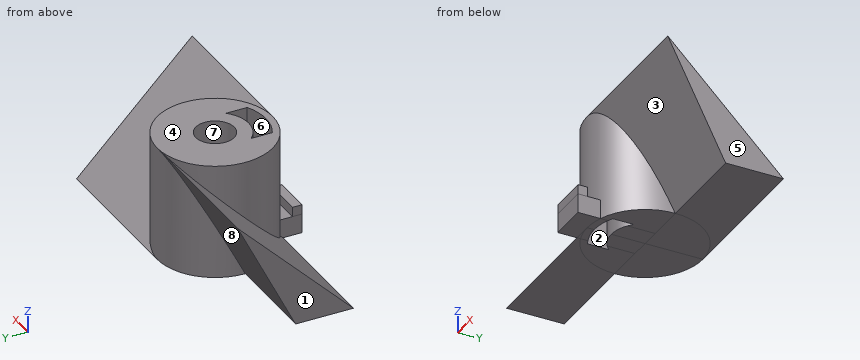
from build123d import *
from build123d import SkipClean  # not in build123d's __all__

# Parameters (mm, degrees)
F0_R      = 7.62
F1_DEPTH  = 15.24
F3_DEPTH  = 20.32
F5_COUNT  = 2
F6_W      = 5.0799995622
F6_H      = 2.54
F7_DEPTH  = 10.16
F8_W      = 5.0799995622
F8_H      = 1.27
F9_DEPTH  = 1.27
F10_R     = 2.54
F11_DEPTH = 13.97
F13_DEPTH = 25.4


with BuildPart() as f1:
    # F0 (on Top) → F1 (new body)
    with BuildSketch(Plane.XY):
        Circle(F0_R)
    extrude(amount=F1_DEPTH)



with BuildPart() as f3:
    # F2 (on Right) → F3 (new body)
    with BuildSketch(Plane.YZ):
        Polygon((-7.62, 15.24), (0, 0), (7.62, 0), align=None)
    extrude(amount=F3_DEPTH)


with BuildPart() as f1_1:
    add(f1.part, clean=False)

    with SkipClean():  # cleaning this boolean's faces spoils the solid; the shape is the same uncleaned
        add(f3.part)  # F5 merges F3
    # F5: F3 ×2 about axis
    f5_axis = Axis((0, 0, 17.5851359963), (0, 0, 1))
    with SkipClean():  # cleaning this boolean's faces spoils the solid; the shape is the same uncleaned
        for i in range(1, F5_COUNT):
            add(f3.part.rotate(f5_axis, i * 360 / F5_COUNT), clean=False)

    # F6 (on Front) → F7 (join)
    with BuildSketch(Plane.XZ):
        with Locations((0, 1.27)):
            Rectangle(F6_W, F6_H)
    with SkipClean():  # cleaning this boolean's faces spoils the solid; the shape is the same uncleaned
        extrude(amount=F7_DEPTH)

    # F8 (on face) → F9 (join)
    with BuildSketch(Plane.XY.offset(2.54)):
        with Locations((0, -9.525)):
            Rectangle(F8_W, F8_H)
    with SkipClean():  # cleaning this boolean's faces spoils the solid; the shape is the same uncleaned
        extrude(amount=F9_DEPTH)

    # F10 (on face) → F11 (cut)
    with BuildSketch(Plane.XY.offset(15.24)):
        Circle(F10_R)
    with SkipClean():  # cleaning this boolean's faces spoils the solid; the shape is the same uncleaned
        extrude(amount=-F11_DEPTH, mode=Mode.SUBTRACT)

    # F12 (on face) → F13 (cut)
    with BuildSketch(Plane.XY.offset(15.24)):
        with BuildLine():
            ThreePointArc((3.175, -3.1108519733), (0, -4.445), (-3.175, -3.1108519733))
            Line((-3.175, -3.1108519733), (-3.175, -5.9048519733))
            ThreePointArc((-3.175, -5.9048519733), (0, -6.7043196394), (3.175, -5.9048519733))
            Line((3.175, -5.9048519733), (3.175, -3.1108519733))
        make_face()
    with SkipClean():  # cleaning this boolean's faces spoils the solid; the shape is the same uncleaned
        extrude(amount=-F13_DEPTH, mode=Mode.SUBTRACT)


solid = f1_1.part
Work out the finished part from the listing and answer in its coordinate system (mm). Face numbers are marked on the shaded views. A direction names the side the tool comes from. Round coordinates to 2 decimals unless told otherwise and drop trailing zeros. Loops run counter-clockwise (first coordinate to the right, second up) from the corner with the lowest first, then second, coordinate; pieces in that order, holes last. Notation, with made-up numbers: M 80.5,-24.75 L 118.5,-24.75 A21 cw 118.5,7.25 Z; hole C 8.25,-30 d7. An arc over 180 degrees is marked long. One line per question, with ' | ' between items. Start each with the question number.
(1) A cutting plane is placed at C-C on y = 5.75. Write down the section's boundary in (x, z).
(2) A cutting plane is placed at B-B on z = 11. Write down the section's boundary in (x, y) (3 decimals).
(3) Flat-ended cylindrical pins translate along their axes: pin 1 Ø4 at (x, y) = (0, 0) entering from +Z; pin 2 Ø2 at (y, z) = (-5, 9) entering from -X; pin 3 Ø1.4 at (x, y) = (0, -9.5) entering from +Z. Find the tip coordinate at first contact, or state that the pin passes through.
(4) A tool of negligible diameter and unlimited length cuts with its end or side. For the marked faces 4, 5, 6, 7 and 8, from which of +Z, -Z, +X, -X, +Y, -Y can it reach the whole face along a straight path? Write none if from no direction.
(5) For a pull along Y with two mould halves and no side action, classify the marked faces 1, 2 and 3 as released by +Y, released by -Y, zero draft, split by the parting line, or undercut.
(6) Find the intervals of material crossed by line 1 (Y direction, x = 0, z = 4.5) (3 decimals); line 2 (Y direction, x = 0.5, z = 3.5); line 3 (X direction, y = -5.25, z = 8.5) (3 decimals), in increasing order.
(7) A cutting plane is placed at A-A on x = -2. Write down the section's boundary in (y, z), plus the area to 3 significant figures.
(8) A cutting plane is placed at D-D on x = 12. Write down the section's boundary in (y, z).
Geometry check:
1) outline: M -20.32,11.5 L -5,11.5 L -5,0 L 20.32,0 L 20.32,1.87 L 5,1.87 L 5,15.24 L -5,15.24 L -5,13.37 L -20.32,13.37 Z
2) outline: M -20.32,3.38 L -6.829,3.38 A7.62 ccw 5.274,-5.5 L 20.32,-5.5 L 20.32,-3.38 L 6.829,-3.38 A7.62 ccw -5.274,5.5 L -20.32,5.5 Z; hole M -3.175,-5.905 A6.704 ccw 3.175,-5.905 L 3.175,-3.111 A4.445 cw -3.175,-3.111 Z; hole C 0,0 d5.08
3) pin 1: stops at z = 1.27 | pin 2: stops at x = -6.49 | pin 3: stops at z = 3.81
4) face 4: +Z, +X, -X, +Y, -Y | face 5: +Z, -Z, +X, +Y, -Y | face 6: +Z, -Z | face 7: +Z | face 8: -Z, -X, +Y
5) face 1: zero draft | face 2: undercut | face 3: released by -Y
6) line 1: y = -7.62 to -6.704, -4.445 to -2.54, 2.54 to 7.62 | line 2: y = -10.16 to -8.89, -7.6 to -6.69, -4.42 to -2.49, 2.49 to 7.6 | line 3: x = -5.523 to -3.175, 3.175 to 5.523
7) outline: M -10.16,0 L -6.4,0 L -6.4,15.24 L -7.35,15.24 L -7.35,2.54 L -8.89,2.54 L -8.89,3.81 L -10.16,3.81 Z; M -3.97,0 L 7.35,0 L 7.35,14.71 L 7.62,15.24 L 7.35,14.97 L 7.35,15.24 L 1.57,15.24 L 1.57,1.27 L -1.57,1.27 L -1.57,15.24 L -3.97,15.24 Z | area: 152 mm²
8) outline: M -7.62,15.24 L 0,0 L 7.62,0 Z
